For this review, take the finished solid that the model builds, in its own axes (mm). A direction names the side the tool comes from. Round coordinates to 2 decimals unless told otherwise and drop trailing zeros. Order: outer loops, then holes, each group sorted by start corner. A loop starts at its lowest first (then second) coordinate and runs counter-clockwise, first axis right, second up. Notation, with made-up numbers: M 89,-28 L 145,-28 A23 cw 145,5 Z; hole C 16,71 d8. An arc over 180 degrees is marked long. Answer as a JSON object with one key per item and string values.
Autodesk Inventor part; units mm, degrees
ref_plane "YZ Plane" through (0, 0, 0) normal (1, 0, 0) x (0, 1, 0)
ref_plane "XZ Plane" through (0, 0, 0) normal (0, 1, 0) x (-1, 0, 0)
ref_plane "XY Plane" through (0, 0, 0) normal (0, 0, 1) x (1, 0, 0)
sketch "Sketch1" plane through (0, 0, 0) normal (0, 0, 1) x (1, 0, 0)
  line L0 (8, -9.5) -> (-8, -9.5)
  line L1 (-8, -9.5) -> (-8, 9.5)
  line L2 (-8, 9.5) -> (8, 9.5)
  line L3 (8, 9.5) -> (8, -9.5)
  line L4 (8, -9.5) -> (-8, 9.5) construction
  line L5 (-8, -9.5) -> (8, 9.5) construction
  circle A0 centre (-5, 6.5) radius 1.5
  circle A1 centre (5, 6.5) radius 1.5
  circle A2 centre (-6.35, -7.9) radius 0.5
  line L6 (0, 9.5) -> (0, -9.5) construction
  circle A3 centre (-3.81, -7.9) radius 0.5
  circle A4 centre (-1.27, -7.9) radius 0.5
  circle A5 centre (1.27, -7.9) radius 0.5
  circle A6 centre (3.81, -7.9) radius 0.5
  circle A7 centre (6.35, -7.9) radius 0.5
  point P0 (0, 0)
  dimension "d0" = 16
  dimension "d1" = 19
  dimension "d3" = 3
  dimension "d4" = 1
  dimension "d5" = 3
  dimension "d6" = 3
  dimension "d7" = 1.6
  dimension "d10" = 2.54
extrude "Extrusion1" add sketch "Sketch1" along normal blind 1.6
sketch "Sketch2" plane through (0, 0, 0) normal (0, 0, -1) x (-1, 0, 0)
  line L0 (2.55, -1) -> (-2.55, -1)
  line L1 (-2.55, -1) -> (-2.55, 2.8)
  line L2 (-2.55, 2.8) -> (2.55, 2.8)
  line L3 (2.55, 2.8) -> (2.55, -1)
  line L4 (2.55, -1) -> (-2.55, 2.8) construction
  line L5 (-2.55, -1) -> (2.55, 2.8) construction
  line L6 (-8, 9.5) -> (8, 9.5)
  point P0 (0, 0)
  point P1 (0, 0.9)
  point P2 (0, 0.9)
  dimension "d17" = 5.1
  dimension "d18" = 3.8
  dimension "d19" = 10.5
extrude "Extrusion2" add sketch "Sketch2" along normal blind 1.5
chamfer "Chamfer1" distance 0.3 angle 45 2 edges at (0, -1, -1.5) (0, 2.8, -1.5)
sketch "Sketch3" plane through (0, 0, 0) normal (0, 0, -1) x (-1, 0, 0)
  line L0 (-8.0252, -9.5) -> (-8.0252, 9.5) construction
  line L1 (-8.0252, 9.5) -> (7.8645, 9.5) construction
  line L2 (7.8645, 9.5) -> (7.8645, -9.5) construction
  line L3 (7.8645, -9.5) -> (-8.0252, -9.5) construction
  line L4 (8, -9.5) -> (-8, -9.5)
  line L5 (-8, 9.5) -> (8, 9.5)
  point P0 (0, 0)
properties part number "CAN_transceiver"
1) For L1, parallel to X at y = 6.25, z = 1.2; L2, parallel to Y at x = 4, z = 0.55; L3, parallel to Y at x = 5, z = 0.6, list the stretches that pass through material, from the lowest coordinate up.
Geometry check:
{"L1": "x = -8 to -6.48, -3.52 to 3.52, 6.48 to 8", "L2": "y = -9.5 to -8.36, -7.44 to 5.38, 7.62 to 9.5", "L3": "y = -9.5 to 5, 8 to 9.5"}
2) Add section C-C on z = 0.7. State how many separate pieces and enclosed holes the cut face has, and give its area (3 significant figures).
Geometry check:
{"separate pieces": "1", "enclosed holes": "8", "area": "285 mm²"}
3) Machinability: for faces 1 (the flat face through (0, 2.8, -1)), 2 (the flat face through (0, -1, -1)), 3 (the flat face through (0, 0, 1.6)), which of the approach directions +Z, -Z, +X, -X, +Y, -Y give a long, thin tool a straight path to every point of the face, cutting with its end or side? Answer none if there is none.
Geometry check:
{"face 1": "-Z, +X, -X, +Y", "face 2": "-Z, +X, -X, -Y", "face 3": "+Z, +X, -X, +Y, -Y"}
4) Insertion check: P1, Ø0.8, axis at y = 1.5, z = -0.5, coming from the +X side; P2, Ø1.5, axis at x = -0.5, y = -3.5, coming from the -Z side; P3, Ø0.6, axis at x = -1, z = -1, coming from the -Y side. Each pin has a flat end and moves straight along its axis. Give the tip position at first contact, or say it passes through.
Geometry check:
{"P1": "stops at x = 2.55", "P2": "stops at z = 0", "P3": "stops at y = -1"}
5) Mouldability with a two-part tool opening along X and no side actions: class faces 4 (the cylindrical face through (-4.21, -7.6, 0.79)), 5 (the flat face through (0, -9.5, 1)), 6 (the flat face through (8, 0, 1)), 7 (the flat face through (-2.55, 1, -1)) as +X half, -X half, draft (parallel to the pull), parting line (faces both ways), or undercut.
Geometry check:
{"face 4": "undercut", "face 5": "draft", "face 6": "+X half", "face 7": "-X half"}
6) Add section D-D on y = 0.25. State the section outline as (x, z) points, and give its area (4 significant figures).
Geometry check:
{"outline": "M -8,0 L -2.55,0 L -2.55,-1.5 L 2.55,-1.5 L 2.55,0 L 8,0 L 8,1.6 L -8,1.6 Z", "area": "33.25 mm²"}
7) Add section A-A on y = 6.5. State the section outline as (x, z) points, and give its area (3 significant figures).
Geometry check:
{"outline": "M -8,0 L -6.5,0 L -6.5,1.6 L -8,1.6 Z; M -3.5,0 L 3.5,0 L 3.5,1.6 L -3.5,1.6 Z; M 6.5,0 L 8,0 L 8,1.6 L 6.5,1.6 Z", "area": "16.0 mm²"}
8) Add section B-B on x = 1.27. State the section outline as (y, z) points, and give its area (3 significant figures).
Geometry check:
{"outline": "M -9.5,0 L -8.4,0 L -8.4,1.6 L -9.5,1.6 Z; M -7.4,0 L -1,0 L -1,-1.2 L -0.7,-1.5 L 2.5,-1.5 L 2.8,-1.2 L 2.8,0 L 9.5,0 L 9.5,1.6 L -7.4,1.6 Z", "area": "34.4 mm²"}
